```python
from build123d import *

# Parameters (mm, degrees)
SKETCH_1_R          = 2.5
SKETCH_1_R_2        = 2.45
SKETCH_1_R_3        = 1.85
SKETCH_1_W          = 48
SKETCH_1_H          = 40
EXTRUDE_1_DEPTH     = 3
SKETCH_2_W          = 20
SKETCH_2_H          = 35
CUT_EXTRUDE_1_DEPTH = 10


with BuildPart() as part:
    # 草图1 → 凸台-拉伸1 (new body)
    # profile 1 of 5: a face of its own
    with BuildSketch(Plane(origin=(0, 0, 0), x_dir=(1, 0, 0), z_dir=(0, 1, 0))):
        with BuildLine():
            Line((8, -30), (8, -70))
            Line((8, -70), (40, -70))
            Line((40, -70), (40, 60))
            Line((40, 60), (32.5, 60))
            ThreePointArc((32.5, 60), (28.232233047, 58.232233047), (30, 62.5))
            Line((30, 62.5), (30, 70))
            Line((30, 70), (8, 70))
            Line((8, 70), (8, 30))
            Line((8, 30), (-40, 30))
            Line((-40, 30), (-40, -30))
            Line((-40, -30), (8, -30))
        make_face()
        with Locations(Location((30, -60, 0), (0, 0, 270))):
            Circle(SKETCH_1_R, mode=Mode.SUBTRACT)
        with Locations(Location((30, 0, 0), (0, 0, 270))):
            Circle(SKETCH_1_R, mode=Mode.SUBTRACT)
    # profile 2 of 5: a face of its own
    with BuildSketch(Plane(origin=(0, 0, 0), x_dir=(1, 0, 0), z_dir=(0, 1, 0))):
        with BuildLine():
            Line((32.5, 60), (40, 60))
            Line((40, 60), (40, 70))
            Line((40, 70), (30, 70))
            Line((30, 70), (30, 62.5))
            ThreePointArc((30, 62.5), (31.767766953, 61.767766953), (32.5, 60))
        make_face()
    # profile 3 of 5: a face of its own
    with BuildSketch(Plane(origin=(0, 0, 0), x_dir=(1, 0, 0), z_dir=(0, 1, 0))):
        with BuildLine():
            Line((-40, 61.45), (-40, 30))
            Line((-40, 30), (8, 30))
            Line((8, 30), (8, 70))
            Line((8, 70), (-30, 70))
            Line((-30, 70), (-30, 63.3))
            ThreePointArc((-30, 63.3), (-28.691852455, 62.758147545), (-28.15, 61.45))
            ThreePointArc((-28.15, 61.45), (-30, 59.6), (-31.85, 61.45))
            Line((-31.85, 61.45), (-40, 61.45))
        make_face()
        with Locations(Location((-31.5, 50, 0), (0, 0, 270))):
            Circle(SKETCH_1_R_2, mode=Mode.SUBTRACT)
        with Locations(Location((-30, 38.55, 0), (0, 0, 270))):
            Circle(SKETCH_1_R_3, mode=Mode.SUBTRACT)
        with Locations(Location((-2, 38.55, 0), (0, 0, 270))):
            Circle(SKETCH_1_R_3, mode=Mode.SUBTRACT)
        with Locations(Location((-0.5, 50, 0), (0, 0, 270))):
            Circle(SKETCH_1_R_2, mode=Mode.SUBTRACT)
        with Locations(Location((-2, 61.45, 0), (0, 0, 270))):
            Circle(SKETCH_1_R_3, mode=Mode.SUBTRACT)
    # profile 4 of 5: a face of its own
    with BuildSketch(Plane(origin=(0, 0, 0), x_dir=(1, 0, 0), z_dir=(0, 1, 0))):
        with BuildLine():
            Line((-40, 70), (-40, 61.45))
            Line((-40, 61.45), (-31.85, 61.45))
            ThreePointArc((-31.85, 61.45), (-31.308147545, 62.758147545), (-30, 63.3))
            Line((-30, 63.3), (-30, 70))
            Line((-30, 70), (-40, 70))
        make_face()
    # profile 5 of 5: a face of its own
    with BuildSketch(Plane(origin=(0, 0, 0), x_dir=(1, 0, 0), z_dir=(0, 1, 0))):
        with Locations((-16, -50)):
            Rectangle(SKETCH_1_W, SKETCH_1_H)
        with Locations(Location((-30, -61.45, 0), (0, 0, 270))):
            Circle(SKETCH_1_R_3, mode=Mode.SUBTRACT)
        with Locations(Location((-31.5, -50, 0), (0, 0, 270))):
            Circle(SKETCH_1_R_2, mode=Mode.SUBTRACT)
        with Locations(Location((-30, -38.55, 0), (0, 0, 270))):
            Circle(SKETCH_1_R_3, mode=Mode.SUBTRACT)
        with Locations(Location((-2, -61.45, 0), (0, 0, 270))):
            Circle(SKETCH_1_R_3, mode=Mode.SUBTRACT)
        with Locations(Location((-0.5, -50, 0), (0, 0, 270))):
            Circle(SKETCH_1_R_2, mode=Mode.SUBTRACT)
        with Locations(Location((-2, -38.55, 0), (0, 0, 270))):
            Circle(SKETCH_1_R_3, mode=Mode.SUBTRACT)
    extrude(amount=EXTRUDE_1_DEPTH)

    # 草图2 → 切除-拉伸1 (cut)
    with BuildSketch(Plane(origin=(0, 3, 0), x_dir=(1, 0, 0), z_dir=(0, 1, 0))):
        with Locations((14, 49.275)):
            Rectangle(SKETCH_2_W, SKETCH_2_H)
        with Locations((14, -49.275)):
            Rectangle(SKETCH_2_W, SKETCH_2_H)
    extrude(amount=-CUT_EXTRUDE_1_DEPTH, mode=Mode.SUBTRACT)


solid = part.part
```
Geometry check sheet. Reference: the model listing, model coordinates, mm. A direction names the side the tool comes from. Give positions to 0.01 mm unless a question says otherwise; leave off trailing zeros. Loops run counter-clockwise (first coordinate to the right, second up) from the corner with the lowest first, then second, coordinate; pieces in that order, holes last. Notation, with made-up numbers: M 50,61 L 96,61 A10 cw 96,66 Z; hole C 37.25,26.25 d9. An arc over 180 degrees is marked long. Answer as CSV lines item,"result".
Item 1: Access from +Z, -Z, +X, -X, +Y, -Y to the whole of each face (thin tool, end or side, straight path). Record for faces 1 (the flat face through (4, 2, 50)), 2 (the flat face through (-1, 1, 70)).
Values:
face 1,"+Y, -Y"
face 2,"+Z, +X, -X, +Y, -Y"
Item 2: Material ranges on line 1 (Z direction, x = 19, y = 0.45) (3 decimals); line 2 (X direction, y = 2, z = -50); line 3 (X direction, y = 1.7, z = -38.55), recorded low to high.
Values:
line 1,"z = -70 to -66.775, -31.775 to 31.775, 66.775 to 70"
line 2,"x = -40 to -33.95, -29.05 to -2.95, 1.95 to 4, 24 to 40"
line 3,"x = -40 to -31.85, -28.15 to -3.85, -0.15 to 4, 24 to 40"
Item 3: Cross-section at B-B on y = 1.9. Count the separate pieces of the cut face and the enclosed holes in it, and give its area (3 significant figures).
Values:
separate pieces,"1"
enclosed holes,"17"
area,"9,580 mm²"
Item 4: Depth check by flat-ended pin: P1, Ø3, axis at x = -30, z = -38.55, coming from the -Y side. Enter the tip coordinate at first touch or a pass-through.
Values:
P1,"passes through"
Item 5: Cross-section at C-C on z = 34.5. Record the cut outline in (x, y), and give its area (3 significant figures).
Values:
outline,"M -40,0 L 4,0 L 4,3 L -40,3 Z; M 24,0 L 40,0 L 40,3 L 24,3 Z"
area,"180 mm²"
Item 6: Cross-section at D-D on z = -38.55. Record the cut outline in (x, y), and give its area (3 significant figures).
Values:
outline,"M -40,0 L -31.85,0 L -31.85,3 L -40,3 Z; M -28.15,0 L -3.85,0 L -3.85,3 L -28.15,3 Z; M -0.15,0 L 4,0 L 4,3 L -0.15,3 Z; M 24,0 L 40,0 L 40,3 L 24,3 Z"
area,"158 mm²"
Item 7: Release check for a two-part mould opening along X. For faces 3 (the flat face through (-40, 1, 1)), 4 (the cylindrical face through (-1.4, 1.5, -59.7)), 5 (the flat face through (40, 1, 1)) record: pulls with the +X half, pulls with the -X half, needs draft (parallel to the pull), parting line crosses it, or undercut.
Values:
face 3,"pulls with the -X half"
face 4,"undercut"
face 5,"pulls with the +X half"
Item 8: Cross-section at A-A on x = 16.5. Record the cut outline in (y, z) (3 decimals).
Values:
outline,"M 0,-70 L 3,-70 L 3,-66.775 L 0,-66.775 Z; M 0,-31.775 L 3,-31.775 L 3,31.775 L 0,31.775 Z; M 0,66.775 L 3,66.775 L 3,70 L 0,70 Z"
